Model file for the job. Use its own axes, mm. A direction names the side the tool comes from. Give positions to 0.01 mm unless a question says otherwise; leave off trailing zeros. Loops run counter-clockwise (first coordinate to the right, second up) from the corner with the lowest first, then second, coordinate; pieces in that order, holes last. Notation, with made-up numbers: M -9.5,37 L 15.5,37 A25 cw 15.5,69 Z; hole C -17,80.5 d1. An arc over 180 degrees is marked long. Answer in a Markdown table with one row per item.
```python
from build123d import *

# Parameters (mm, degrees)
SKETCH1_R               = 10.9855
BOSS_EXTRUDE1_DEPTH     = 2
SKETCH3_R               = 5
BOSS_EXTRUDE2_DEPTH     = 10
SKETCH2_R               = 2.5
CUT_EXTRUDE1_DEPTH      = 11
CUT_EXTRUDE1_DEPTH_BACK = 3
SKETCH4_R               = 1.5
CUT_EXTRUDE2_DEPTH      = 10


with BuildPart() as part:
    # Sketch1 → Boss-Extrude1 (new body)
    with BuildSketch(Plane(origin=(0, 0, 0), x_dir=(1, 0, 0), z_dir=(0, 1, 0))):
        Circle(SKETCH1_R)
    extrude(amount=BOSS_EXTRUDE1_DEPTH)

    # Sketch3 → Boss-Extrude2 (add)
    with BuildSketch(Plane(origin=(0, 2, 0), x_dir=(1, 0, 0), z_dir=(0, 1, 0))):
        Circle(SKETCH3_R)
    extrude(amount=BOSS_EXTRUDE2_DEPTH)

    # Sketch2 → Cut-Extrude1 (cut, two sides)
    with BuildSketch(Plane(origin=(0, 2, 0), x_dir=(1, 0, 0), z_dir=(0, 1, 0))) as cut_extrude1_sk:
        Circle(SKETCH2_R)
    extrude(amount=CUT_EXTRUDE1_DEPTH, mode=Mode.SUBTRACT)
    extrude(cut_extrude1_sk.sketch, amount=-CUT_EXTRUDE1_DEPTH_BACK, mode=Mode.SUBTRACT)

    # Sketch4 → Cut-Extrude2 (cut)
    with BuildSketch(Plane(origin=(0, 2, 0), x_dir=(1, 0, 0), z_dir=(0, 1, 0))):
        with Locations((8, 0)):
            Circle(SKETCH4_R)
        with Locations((0, -8)):
            Circle(SKETCH4_R)
        with Locations((-8, 0)):
            Circle(SKETCH4_R)
        with Locations((0, 8)):
            Circle(SKETCH4_R)
    extrude(amount=-CUT_EXTRUDE2_DEPTH, mode=Mode.SUBTRACT)


solid = part.part
```
(1) Wall check: L1, parallel to Z at x = 0, y = 0.45; L2, parallel to Z at x = 0, y = 4.25. Give the ranges that are in metal, low to high.
Established:
| item | result |
|---|---|
| L1 | z = -10.99 to -9.5, -6.5 to -2.5, 2.5 to 6.5, 9.5 to 10.99 |
| L2 | z = -5 to -2.5, 2.5 to 5 |
(2) Saw through at D-D, the plane x = 8. Give the cut face in (y, z), and give its area (3 significant figures).
Established:
| item | result |
|---|---|
| outline | M 0,-7.53 L 2,-7.53 L 2,-1.5 L 0,-1.5 Z; M 0,1.5 L 2,1.5 L 2,7.53 L 0,7.53 Z |
| area | 24.1 mm2 |
(3) Flat gauge pins, fed straight in: P1, Ø4, axis at x = 0, z = 0, coming from the +Y side; P2, Ø3, axis at y = 7, z = 6, coming from the +X side; P3, Ø8, axis at x = -2.5, z = 7, coming from the -Y side; P4, Ø6, axis at y = 8.5, z = -1, coming from the +X side. Where does each tip first touch, or does it go through?
Established:
| item | result |
|---|---|
| P1 | passes through |
| P2 | stops at x = 2.18 |
| P3 | stops at y = 0 |
| P4 | stops at x = 5 |
(4) Mould opens along Z. For faces 1 (the flat face through (2, 12, 2)), 2 (the cylindrical face through (-0.325, 1.014, 9.464)), 3 (the cylindrical face through (-9.5, 1.01, -0.07)), 4 (the cylindrical face through (-1.08, 6.93, 4.88)) say: pulls with the +Z half, pulls with the -Z half, needs draft (parallel to the pull), parting line crosses it, or undercut.
Established:
| item | result |
|---|---|
| face 1 | needs draft |
| face 2 | undercut |
| face 3 | undercut |
| face 4 | parting line crosses it |
(5) Saw through at B-B, the plane z = 0. Give the cut face in (x, y).
Established:
| item | result |
|---|---|
| outline | M -10.99,0 L -9.5,0 L -9.5,2 L -10.99,2 Z; M -6.5,0 L -2.5,0 L -2.5,12 L -5,12 L -5,2 L -6.5,2 Z; M 2.5,0 L 6.5,0 L 6.5,2 L 5,2 L 5,12 L 2.5,12 Z; M 9.5,0 L 10.99,0 L 10.99,2 L 9.5,2 Z |
(6) Which spindle directions (+Z, -Z, +X, -X, +Y, -Y) get a long thin tool onto all of the face, cutting with end or side? Do faces 5 (the cylindrical face through (-0.325, 1.014, -6.536)), 6 (the flat face through (5, 2, 2)). Say none if no direction does.
Established:
| item | result |
|---|---|
| face 5 | +Y, -Y |
| face 6 | +Y |
(7) Saw through at A-A, the plane x = 0. Give the cut face in (y, z), and give its area (3 significant figures).
Established:
| item | result |
|---|---|
| outline | M 0,-10.99 L 2,-10.99 L 2,-9.5 L 0,-9.5 Z; M 0,-6.5 L 2,-6.5 L 2,-5 L 12,-5 L 12,-2.5 L 0,-2.5 Z; M 0,2.5 L 12,2.5 L 12,5 L 2,5 L 2,6.5 L 0,6.5 Z; M 0,9.5 L 2,9.5 L 2,10.99 L 0,10.99 Z |
| area | 71.9 mm2 |
(8) Saw through at C-C, the plane z = -8. Give the cut face in (x, y), and give its area (3 significant figures).
Established:
| item | result |
|---|---|
| outline | M -7.53,0 L -1.5,0 L -1.5,2 L -7.53,2 Z; M 1.5,0 L 7.53,0 L 7.53,2 L 1.5,2 Z |
| area | 24.1 mm2 |
